For this review, take the finished solid that the model builds, in its own axes (mm). Face numbers are marked on the shaded views. A direction names the side the tool comes from. Round coordinates to 2 decimals unless told otherwise and drop trailing zeros. Order: outer loops, then holes, each group sorted by start corner. A loop starts at its lowest first (then second) coordinate and runs counter-clockwise, first axis right, second up. Notation, with made-up numbers: M 53.5,48 L 71.5,48 A9 cw 71.5,64 Z; hole C -37.5,-24.75 d7. An arc over 180 degrees is marked long. Use a Markdown table: item, result.
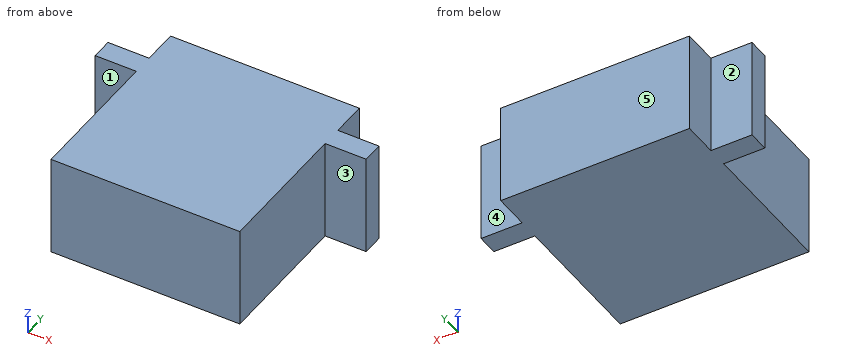
Autodesk Inventor part; units mm, degrees
sketch "Skizze1" plane through (0, 0, 0) normal (0, 0, 1) x (1, 0, 0)
  line L0 (-11.25, 0) -> (11.25, 0)
  line L1 (11.25, 0) -> (11.25, 16.7)
  line L2 (11.25, 16.7) -> (-11.25, 16.7)
  line L3 (-11.25, 16.7) -> (-11.25, 0)
  line L4 (0, -4.68) -> (0, 28.08)
  line L5 (-11.25, 16.7) -> (-16.15, 16.7)
  line L6 (-16.15, 16.7) -> (-16.15, 19.2)
  line L7 (-16.15, 19.2) -> (-11.25, 19.2)
  line L8 (-11.25, 19.2) -> (-11.25, 23.4)
  line L9 (-11.25, 23.4) -> (0, 23.4)
  line L10 (11.25, 16.7) -> (16.15, 16.7)
  line L11 (16.15, 16.7) -> (16.15, 19.2)
  line L12 (16.15, 19.2) -> (11.25, 19.2)
  line L13 (11.25, 19.2) -> (11.25, 23.4)
  line L14 (11.25, 23.4) -> (0, 23.4)
  point P0 (0, 0)
  dimension "d0" = 22.5
  dimension "d1" = 16.7
  dimension "d2" = 4.9
  dimension "d3" = 2.5
  dimension "d4" = 4.2
  dimension "d5" = 22.5
extrude "Extrusion1" add sketch "Skizze1" along normal mid plane 12.1
properties part number "Motortest"
Q1. Machinability: for the marked faces 1, 2, 3, 4 and 5, which of the approach directions +Z, -Z, +X, -X, +Y, -Y give a long, thin tool a straight path to every point of the face, cutting with its end or side? Answer none if there is none.
Determined:
| item | result |
|---|---|
| face 1 | +Z, -Z, -X, -Y |
| face 2 | +Z, -Z, -X, +Y |
| face 3 | +Z, -Z, +X, -Y |
| face 4 | +Z, -Z, +X, +Y |
| face 5 | +Z, -Z, +X, -X, +Y |
Q2. Wall thickness on line 1 along Y through (x, z) = (-13.5, 1); line 2 along X through (y, z) = (1.5, 4.75): over which ranges is each line inside the solid? List them lowest first. Write a range as [from, to].
Determined:
| item | result |
|---|---|
| line 1 | y = [16.7, 19.2] |
| line 2 | x = [-11.25, 11.25] |
Q3. Add section A-A (z = 1.5). Write out the cut boundary in (x, y).
Determined:
| item | result |
|---|---|
| outline | M -16.15,16.7 L -11.25,16.7 L -11.25,0 L 11.25,0 L 11.25,16.7 L 16.15,16.7 L 16.15,19.2 L 11.25,19.2 L 11.25,23.4 L -11.25,23.4 L -11.25,19.2 L -16.15,19.2 Z |
Q4. Clearance check with flat-ended pins moving along their axes: pin 1 (3.5 mm diameter, centred on y = 21.5, z = -0.5, fed in from -X); pin 2 (1.5 mm diameter, centred on x = -13, z = 0.5, fed in from -Y); pin 3 (1.5 mm diameter, centred on x = 13, z = 2, fed in from +Y). State where each tip first meets the part, or that it passes through.
Determined:
| item | result |
|---|---|
| pin 1 | stops at x = -11.25 |
| pin 2 | stops at y = 16.7 |
| pin 3 | stops at y = 19.2 |
Q5. Add section C-C (x = 12). Write out the cut boundary in (y, z).
Determined:
| item | result |
|---|---|
| outline | M 16.7,-6.05 L 19.2,-6.05 L 19.2,6.05 L 16.7,6.05 Z |
Q6. Add section B-B (y = 22). Write out the cut boundary in (x, z), then the cut area to 3 significant figures.
Determined:
| item | result |
|---|---|
| outline | M -11.25,-6.05 L 11.25,-6.05 L 11.25,6.05 L -11.25,6.05 Z |
| area | 272 mm^2 |
